Check sheet for the modelled part. Datum: model origin and axes. Units: mm. Face numbers are marked on the shaded views. A direction names the side the tool comes from. Give positions to 0.01 mm unless a question says otherwise; leave off trailing zeros. Write each loop counter-clockwise with the first axis right and the second up, starting at its lowest first coordinate (ties: lowest second). Pieces come first, ordered by that corner, then holes. Notation, with made-up numbers: M 87,64 L 126,64 A18 ccw 126,97 Z; hole C 15,52.5 d5. An arc over 180 degrees is marked long. Write item = value, one per line. Start each with the question number.
1) Access from +Z, -Z, +X, -X, +Y, -Y to the whole of each face (thin tool, end or side, straight path). Record for the marked faces 4, 5 and 6.
2) Go/stop test with flat-tipped pins: pin 1 (4 mm diameter, centred on x = 2.5, y = 5.5, fed in from +Z); pin 2 (0.6 mm diameter, centred on y = -0.5, z = 2.5, fed in from -X); pin 3 (4 mm diameter, centred on x = -3, z = 5.5, fed in from -Y). Record where each tip stops, or that it passes through.
3) Cross-section at A-A, the plane x = 0. Record the cut outline in (y, z), plus the area to 3 significant figures.
4) Cross-section at C-C, the plane y = 2.75. Record the cut outline in (x, z).
5) Cross-section at B-B, the plane z = 7. Record the cut outline in (x, y), plus the area to 3 significant figures.
6) Scan lines: line 1 along Y through (x, z) = (-3.75, 3.5); line 2 along Y through (x, z) = (-0.25, 3.25); line 3 along Y through (x, z) = (-3.5, 8.25). Record each from-to range of solid material in increasing order. Write a range as [from, to].
7) Mould release check, pull along X, two halves, no side actions. Record for the marked faces 1, 2 and 3: released by +X, released by -X, zero draft, split by the parting line, or undercut.
8) Cross-section at D-D, the plane z = 2. Record the cut outline in (x, y), plus the area to 3 significant figures.
```python
from build123d import *

# Parameters (mm, degrees)
CUT_EXTRUDE1_START  = -6.35
CUT_EXTRUDE1_DEPTH  = 6.35
SKETCH3_R           = 1.190625
CUT_EXTRUDE2_DEPTH  = 3.048
SKETCH4_R           = 0.762
SKETCH4_R_2         = 0.8255
BOSS_EXTRUDE1_DEPTH = 0.79375
CUT_EXTRUDE3_START  = -1.5875
SKETCH6_R           = 0.8255
CUT_EXTRUDE3_DEPTH  = 1.5875
SKETCH7_W           = 1.5875
SKETCH7_H           = 6.35
BOSS_EXTRUDE2_DEPTH = 0.79375


# Read off the part's stored shape, not the designer's step: Cut-Extrude1
with BuildPart() as part:
    # Sketch1 → Revolve1 (revolve)
    with BuildSketch(Plane.XY):
        Polygon((0, 1.5875), (0, 0), (9.271, 0), (9.271, 6.35), (0, 6.35), (0, 4.7625), (7.6835, 4.7625), (7.6835, 1.5875), align=None)
    revolve(axis=Axis((0, 0, 0), (0, 1, 0)))

    # Cut-Extrude1 outline → Cut-Extrude1 (cut)
    with BuildSketch(Plane(origin=(0, 6.35, 0), x_dir=(1, 0, 0), z_dir=(0, 1, 0)).offset(CUT_EXTRUDE1_START)):
        with BuildLine():
            Line((-9.271, 0), (9.271, 0))
            ThreePointArc((9.271, 0), (0, 9.271), (-9.271, 0))
        make_face()
    extrude(amount=CUT_EXTRUDE1_DEPTH, mode=Mode.SUBTRACT)

    # Sketch3 → Cut-Extrude2 (cut)
    with BuildSketch(Plane.XZ):
        with Locations((5.30225, 0)):
            Circle(SKETCH3_R)
        with Locations((-5.30225, 0)):
            Circle(SKETCH3_R)
    extrude(amount=-CUT_EXTRUDE2_DEPTH, mode=Mode.SUBTRACT)

    # Sketch4 → Boss-Extrude1 (add)
    with BuildSketch(Plane(origin=(0, 0, 0), x_dir=(-1, 0, 0), z_dir=(0, 0, -1))):
        with Locations(Location((-8.382, 5.461, 0), (0, 0, 180))):
            Circle(SKETCH4_R)
        with Locations(Location((-8.382, 0.889, 0), (0, 0, 180))):
            Circle(SKETCH4_R_2)
        with Locations(Location((8.382, 5.461, 0), (0, 0, 180))):
            Circle(SKETCH4_R_2)
        with Locations(Location((8.382, 0.889, 0), (0, 0, 180))):
            Circle(SKETCH4_R)
    extrude(amount=BOSS_EXTRUDE1_DEPTH)

    # Sketch6 → Cut-Extrude3 (cut)
    with BuildSketch(Plane(origin=(0, 0, -0.79375), x_dir=(-1, 0, 0), z_dir=(0, 0, -1)).offset(CUT_EXTRUDE3_START)):
        with Locations((-8.382, 0.889)):
            Circle(SKETCH6_R)
        with Locations((8.382, 5.461)):
            Circle(SKETCH6_R)
    extrude(amount=CUT_EXTRUDE3_DEPTH, mode=Mode.SUBTRACT)

    # Sketch7 → Boss-Extrude2 (add)
    with BuildSketch(Plane.XZ):
        with Locations((0, 3.175)):
            Rectangle(SKETCH7_W, SKETCH7_H)
    extrude(amount=BOSS_EXTRUDE2_DEPTH)


solid = part.part
```
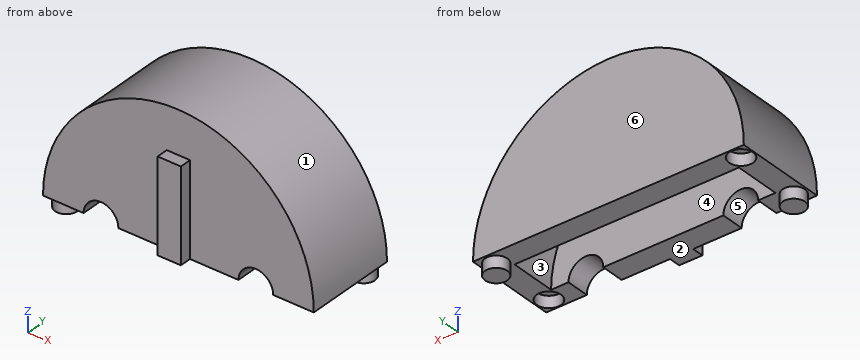
Reply:
q1.face_4 = -Z
q1.face_5 = -Z, -Y
q1.face_6 = +Z, -Z, +X, -X, +Y
q2.pin_1 = 9.26
q2.pin_2 = -0.79
q2.pin_3 = 0
q3.outline = M -0.79,0 L 1.59,0 L 1.59,7.68 L 4.76,7.68 L 4.76,0 L 6.35,0 L 6.35,9.27 L 0,9.27 L 0,6.35 L -0.79,6.35 Z
q3.area = 39.5 mm2
q4.outline = M -9.27,0 L -7.68,0 A7.68 cw 7.68,0 L 9.27,0 A9.27 ccw Z
q5.outline = M -6.08,0 L 6.08,0 L 6.08,6.35 L -6.08,6.35 Z; hole M -3.17,1.59 L 3.17,1.59 L 3.17,4.76 L -3.17,4.76 Z
q5.area = 57.1 mm2
q6.line_1 = [0, 1.59], [4.76, 6.35]
q6.line_2 = [-0.79, 1.59], [4.76, 6.35]
q6.line_3 = [0, 6.35]
q7.face_1 = split by the parting line
q7.face_2 = zero draft
q7.face_3 = undercut
q8.outline = M -9.05,0 L -0.79,0 L -0.79,-0.79 L 0.79,-0.79 L 0.79,0 L 9.05,0 L 9.05,6.35 L -9.05,6.35 Z; hole M -7.42,1.59 L 7.42,1.59 L 7.42,4.76 L -7.42,4.76 Z
q8.area = 69.1 mm2
